Geometry check sheet. Reference: the model listing, model coordinates, mm. A direction names the side the tool comes from. Coordinates: 2 decimals unless noted, no trailing zeros. Order: outer loops, then holes, each group sorted by start corner. A loop starts at its lowest first (then second) coordinate and runs counter-clockwise, first axis right, second up. Notation, with made-up numbers: (70.25, -10) - (108.25, -10) arc R28 cw to (108.25, 10) - close; hole circle Ø7 at (8.5, 17.5). An arc over 180 degrees is marked (long way). Return JSON: item names as keys, results as strings. Group by question number.
Item 1: Gauge pin test, flat ends, axial feed: pin 1 (4 mm diameter, centred on x = -9, y = 32, fed in from -Z); pin 2 (12 mm diameter, centred on y = 35, z = 18.5, fed in from -X); pin 3 (1.1 mm diameter, centred on x = 16, y = 44.5, fed in from +Z). Record the tip position at first contact, or that the pin passes through.
Item 2: Tool access check on faces 5 (the flat face through (0, 25, 22)), 6 (the flat face through (-17, 25, 0)), 7 (the flat face through (0, 5, 0)), 8 (the flat face through (0, 25, -22)). Record the directions out of +Z, -Z, +X, -X, +Y, -Y that give a thin tool (end or side, any length) a straight path to the whole face; none if there is none.
Item 3: Section check A-A on y = 6. Enter the section's corners in (x, z).
Item 4: Scan lines: probe 1 along Z at (x, y) = (-8.5, 39.5); probe 2 along X at (y, z) = (19, 2); probe 3 along X at (y, z) = (40.5, 20.5). Record each from-to range of solid material in increasing order.
Item 5: Draft check along X on faces 1 (the flat face through (0, 25, 20)), 2 (the flat face through (17, 25, 0)), 3 (the flat face through (0, 2, 25)), 4 (the flat face through (0, 25, -20)). Enter one of: pulls with the +X half, pulls with the -X half, needs draft (parallel to the pull), parting line crosses it, or undercut.
Item 6: Section check B-B on x = -7. Enter the section's corners in (y, z).
Item 7: Section check C-C on z = -7.5. Enter the section's corners in (x, y).
Autodesk Inventor part; units mm, degrees
ref_plane "YZ Plane" through (0, 0, 0) normal (1, 0, 0) x (0, 1, 0)
ref_plane "XZ Plane" through (0, 0, 0) normal (0, 1, 0) x (-1, 0, 0)
ref_plane "XY Plane" through (0, 0, 0) normal (0, 0, 1) x (1, 0, 0)
sketch "Sketch1" plane through (0, 0, 0) normal (0, 1, 0) x (-1, 0, 0)
  line L0 (-20, -25) -> (20, -25)
  line L1 (20, -25) -> (20, 25)
  line L2 (20, 25) -> (-20, 25)
  line L3 (-20, 25) -> (-20, -25)
  line L4 (-20, -25) -> (20, 25) construction
  line L5 (20, -25) -> (-20, 25) construction
  point P0 (0, 0)
  dimension "d2" = 40
  dimension "d3" = 50
extrude "Extrusion1" add sketch "Sketch1" along normal blind 5
sketch "Sketch2" plane through (0, 5, 0) normal (0, 1, 0) x (1, 0, 0)
  line L0 (-20, 25) -> (-20, -25)
  line L1 (-20, -25) -> (20, -25)
  line L2 (20, -25) -> (20, 25)
  line L3 (20, 25) -> (-20, 25)
  line L4 (17, 22) -> (-17, 22)
  line L5 (-17, 22) -> (-17, -22)
  line L6 (-17, -22) -> (17, -22)
  line L7 (17, -22) -> (17, 22)
  line L8 (17, 22) -> (-17, -22) construction
  line L9 (-17, 22) -> (17, -22) construction
  line L10 (15, 20) -> (-15, 20)
  line L11 (-15, 20) -> (-15, -20)
  line L12 (-15, -20) -> (15, -20)
  line L13 (15, -20) -> (15, 20)
  line L14 (15, 20) -> (-15, -20) construction
  line L15 (-15, 20) -> (15, -20) construction
  point P0 (0, 0)
  dimension "d6" = 3
  dimension "d7" = 2
  dimension "d52" = 3
  dimension "d53" = 2
extrude "Extrusion2" add sketch "Sketch2" along normal blind 40 contours L7 L6 L5 L4
fillet "Fillet1" radius 1 1 edges at (20, 2.5, 25)
fillet "Fillet2" radius 1 1 edges at (20, 2.5, -25)
fillet "Fillet3" radius 1 1 edges at (-20, 2.5, 25)
fillet "Fillet4" radius 1 1 edges at (-20, 2.5, -25)
fillet "Fillet5" radius 1 1 edges at (-17, 25, 22)
fillet "Fillet6" radius 1 1 edges at (17, 25, 22)
fillet "Fillet7" radius 1 1 edges at (17, 25, -22)
fillet "Fillet8" radius 1 1 edges at (-17, 25, -22)
sketch "Sketch3" plane through (0, 45, 0) normal (0, 1, 0) x (1, 0, 0)
  arc A0 (-16, 22) -> (-17, 21) centre (-16, 21) ccw
  line L0 (-17, 21) -> (-17, -21)
  arc A1 (-17, -21) -> (-16, -22) centre (-16, -21) ccw
  line L1 (-16, -22) -> (16, -22)
  arc A2 (16, -22) -> (17, -21) centre (16, -21) ccw
  line L2 (17, -21) -> (17, 21)
  arc A3 (17, 21) -> (16, 22) centre (16, 21) ccw
  line L3 (16, 22) -> (-16, 22)
  line L4 (15, 20) -> (15, -20)
  line L5 (15, -20) -> (-15, -20)
  line L6 (-15, -20) -> (-15, 20)
  line L7 (-15, 20) -> (15, 20)
  line L8 (-16.5, -15) -> (-15.5, -15)
  line L9 (-15.5, -15) -> (-15.5, 5)
  line L10 (-15.5, 5) -> (-16.5, 5)
  line L11 (-16.5, 5) -> (-16.5, -15)
  line L12 (-16.5, 15) -> (-15.5, 15)
  line L13 (-15.5, 15) -> (-15.5, -5)
  line L14 (-15.5, -5) -> (-16.5, -5)
  line L15 (-16.5, -5) -> (-16.5, 15)
  line L16 (-10, 21.5) -> (10, 21.5)
  line L17 (10, 21.5) -> (10, 20.5)
  line L18 (10, 20.5) -> (-10, 20.5)
  line L19 (-10, 20.5) -> (-10, 21.5)
  line L20 (10, 21.5) -> (-10, 21.5)
  line L21 (-10, 21.5) -> (-10, 20.5)
  line L22 (-10, 20.5) -> (10, 20.5)
  line L23 (10, 20.5) -> (10, 21.5)
  line L24 (15.5, 15) -> (16.5, 15)
  line L25 (16.5, 15) -> (16.5, -5)
  line L26 (16.5, -5) -> (15.5, -5)
  line L27 (15.5, -5) -> (15.5, 15)
  line L28 (15.5, -15) -> (16.5, -15)
  line L29 (16.5, -15) -> (16.5, 5)
  line L30 (16.5, 5) -> (15.5, 5)
  line L31 (15.5, 5) -> (15.5, -15)
  line L32 (10, -20.5) -> (-10, -20.5)
  line L33 (-10, -20.5) -> (-10, -21.5)
  line L34 (-10, -21.5) -> (10, -21.5)
  line L35 (10, -21.5) -> (10, -20.5)
  line L36 (-10, -20.5) -> (10, -20.5)
  line L37 (10, -20.5) -> (10, -21.5)
  line L38 (10, -21.5) -> (-10, -21.5)
  line L39 (-10, -21.5) -> (-10, -20.5)
  point P0 (0, 0)
  point P1 (-16, 15)
  point P2 (-16, -5)
  point P3 (16, 15)
  dimension "d18" = 1
  dimension "d19" = 20
  dimension "d20" = 0.5
  dimension "d21" = 7
  dimension "d22" = 7
  dimension "d23" = 0.5
  dimension "d24" = 1
  dimension "d25" = 20
  dimension "d26" = 20
  dimension "d27" = 1
  dimension "d28" = 0.5
  dimension "d29" = 7
  dimension "d30" = 20
  dimension "d31" = 1
  dimension "d32" = 0.5
  dimension "d33" = 7
  dimension "d34" = 1
  dimension "d35" = 20
  dimension "d36" = 0.5
  dimension "d37" = 7
  dimension "d38" = 1
  dimension "d39" = 20
  dimension "d40" = 7
  dimension "d41" = 0.5
  dimension "d42" = 20
  dimension "d43" = 1
  dimension "d44" = 0.5
  dimension "d45" = 7
  dimension "d46" = 20
  dimension "d47" = 1
  dimension "d48" = 0.5
  dimension "d49" = 7
extrude "Extrusion3" cut sketch "Sketch3" against normal blind 1 contours L11 L14 L9 L8 | L11 L10 L9 L14 | L15 L12 L13 L10 | L16 L17 L18 L19 | L24 L25 L30 L27 | L30 L25 L26 L27 | L26 L29 L28 L31 | L35 L34 L33 L32
properties part number "block_main" material "PC/ABS Plastic"
Computed:
{
 "1": {"pin 1": "stops at z = -22", "pin 2": "stops at x = -17", "pin 3": "stops at z = 22"},
 "2": {"face 5": "+Z, +X, -X, +Y", "face 6": "+Z, -Z, -X, +Y", "face 7": "+Y", "face 8": "-Z, +X, -X, +Y"},
 "3": {"outline": "(-17, -21) arc R1 ccw to (-16, -22) - (16, -22) arc R1 ccw to (17, -21) - (17, 21) arc R1 ccw to (16, 22) - (-16, 22) arc R1 ccw to (-17, 21) - close; hole (-15, -20) - (15, -20) - (15, 20) - (-15, 20) - close"},
 "4": {"probe 1": "z = -22 to -20, 20 to 22", "probe 2": "x = -17 to -15, 15 to 17", "probe 3": "x = -17 to 17"},
 "5": {"face 1": "undercut", "face 2": "pulls with the +X half", "face 3": "needs draft", "face 4": "undercut"},
 "6": {"outline": "(0, -25) - (5, -25) - (5, -22) - (45, -22) - (45, -21.5) - (44, -21.5) - (44, -20.5) - (45, -20.5) - (45, -20) - (5, -20) - (5, 20) - (45, 20) - (45, 20.5) - (44, 20.5) - (44, 21.5) - (45, 21.5) - (45, 22) - (5, 22) - (5, 25) - (0, 25) - close"},
 "7": {"outline": "(-20, 0) - (20, 0) - (20, 5) - (17, 5) - (17, 45) - (16.5, 45) - (16.5, 44) - (15.5, 44) - (15.5, 45) - (15, 45) - (15, 5) - (-15, 5) - (-15, 45) - (-15.5, 45) - (-15.5, 44) - (-16.5, 44) - (-16.5, 45) - (-17, 45) - (-17, 5) - (-20, 5) - close"}
}
